from build123d import *

# Parameters (mm, degrees)
ESQUISSE1_W             = 9.3
ESQUISSE1_H             = 75
BOSS_EXTRU_1_DEPTH      = 6.5
ESQUISSE2_R             = 0.75
ENL_V_MAT_EXTRU_1_DEPTH = 4
ESQUISSE3_W             = 1.2
ESQUISSE3_H             = 67
ENL_V_MAT_EXTRU_2_DEPTH = 4
BOSS_EXTRU_2_DEPTH      = 0.6


with BuildPart() as part:
    # Esquisse1 → Boss.-Extru.1 (new body)
    with BuildSketch(Plane(origin=(0, 0, 0), x_dir=(1, 0, 0), z_dir=(0, 1, 0))):
        Rectangle(ESQUISSE1_W, ESQUISSE1_H)
    extrude(amount=BOSS_EXTRU_1_DEPTH)

    # Esquisse2 → Enlèv. mat.-Extru.1 (cut)
    with BuildSketch(Plane(origin=(0, 6.5, 0), x_dir=(1, 0, 0), z_dir=(0, 1, 0))):
        with Locations(Location((0, 35.5, 0), (0, 0, 270))):
            Circle(ESQUISSE2_R)
        with Locations(Location((0, -35.5, 0), (0, 0, 270))):
            Circle(ESQUISSE2_R)
    extrude(amount=-ENL_V_MAT_EXTRU_1_DEPTH, mode=Mode.SUBTRACT)

    # Esquisse3 → Enlèv. mat.-Extru.2 (cut)
    with BuildSketch(Plane(origin=(0, 6.5, 0), x_dir=(1, 0, 0), z_dir=(0, 1, 0))):
        Rectangle(ESQUISSE3_W, ESQUISSE3_H)
    extrude(amount=-ENL_V_MAT_EXTRU_2_DEPTH, mode=Mode.SUBTRACT)

    # Esquisse4 → Boss.-Extru.2 (add, symmetric)
    with BuildSketch(Plane(origin=(0, 0, 0), x_dir=(0, 0, -1), z_dir=(1, 0, 0))):
        Polygon((-26.491586963, 2.5), (-21.491586963, 2.5), (-21.491586963, 11), (-21.991586963, 11.5), (-21.991586963, 21.5), (-25.991586963, 21.5), (-25.991586963, 11.5), (-26.491586963, 11), align=None)
    extrude(amount=BOSS_EXTRU_2_DEPTH, both=True)


solid = part.part
Verification items for the finished model (mm, model axes). A direction names the side the tool comes from. Give positions to 0.01 mm unless a question says otherwise; leave off trailing zeros. Write each loop counter-clockwise with the first axis right and the second up, starting at its lowest first coordinate (ties: lowest second). Pieces come first, ordered by that corner, then holes. Notation, with made-up numbers: (55.25, -7.5) -> (73.25, -7.5) arc R11 ccw to (73.25, 13.5) -> close; hole circle Ø9 at (-2.75, -20.5). An arc over 180 degrees is marked (long way). Use CSV: the item, a comma, the result in double quotes.
(1) Sectioned sample at B-B (z = -35.5). Record the cut outline in (x, y).
Derived:
outline,"(-4.65, 0) -> (4.65, 0) -> (4.65, 6.5) -> (0.75, 6.5) -> (0.75, 2.5) -> (-0.75, 2.5) -> (-0.75, 6.5) -> (-4.65, 6.5) -> close"
(2) Set-up check for faces 4 (the cylindrical face through (0.225, 4.528, -34.785)), 5 (the flat face through (0, 17, 25.992)), 6 (the flat face through (0.6, 14, 24)): record each of +Z, -Z, +X, -X, +Y, -Y from which the full face is reachable in a straight line by a thin tool's end or side.
Derived:
face 4,"+Y"
face 5,"+Z, +X, -X, +Y"
face 6,"+Z, -Z, +X, +Y"
(3) Go/stop test with flat-tipped pins: pin 1 (1.5 mm diameter, centred on x = -2, z = -28, fed in from +Y); pin 2 (1 mm diameter, centred on x = 0, y = 8.5, fed in from +Z); pin 3 (3 mm diameter, centred on x = -2, y = 16.5, fed in from +Z); pin 4 (2 mm diameter, centred on x = -3, y = 12, fed in from +Z). Record where each tip stops, or that it passes through.
Derived:
pin 1,"stops at y = 6.5"
pin 2,"stops at z = 26.49"
pin 3,"stops at z = 25.99"
pin 4,"passes through"
(4) Sectioned sample at D-D (z = 12). Record the cut outline in (x, y), plus the area to 4 significant figures.
Derived:
outline,"(-4.65, 0) -> (4.65, 0) -> (4.65, 6.5) -> (0.6, 6.5) -> (0.6, 2.5) -> (-0.6, 2.5) -> (-0.6, 6.5) -> (-4.65, 6.5) -> close"
area,"55.65 mm^2"
(5) Release check for a two-part mould opening along X. For faces 1 (the flat face through (0, 2.5, 30)), 2 (the flat face through (-1, 6.5, -1)), 3 (the flat face through (4.65, 3, 1)) record: +X half, -X half, draft (parallel to the pull), parting line (faces both ways), or undercut.
Derived:
face 1,"undercut"
face 2,"draft"
face 3,"+X half"
(6) Sectioned sample at A-A (y = 3.5). Record the cut outline in (x, z).
Derived:
outline,"(-4.65, -37.5) -> (4.65, -37.5) -> (4.65, 37.5) -> (-4.65, 37.5) -> close; hole circle Ø1.5 at (0, -35.5); hole circle Ø1.5 at (0, 35.5); hole (-0.6, -33.5) -> (0.6, -33.5) -> (0.6, 21.49) -> (-0.6, 21.49) -> close; hole (-0.6, 26.49) -> (0.6, 26.49) -> (0.6, 33.5) -> (-0.6, 33.5) -> close"
(7) Sectioned sample at C-C (x = -2). Record the cut outline in (y, z), plus the area to 4 significant figures.
Derived:
outline,"(0, -37.5) -> (6.5, -37.5) -> (6.5, 37.5) -> (0, 37.5) -> close"
area,"487.5 mm^2"
(8) Material ranges on L1, parallel to X at y = 6.25, z = -24; L2, parallel to X at y = 3.9, z = 35.5; L3, parallel to Z at x = -0.25, y = 4.5, recorded low to high.
Derived:
L1,"x = -4.65 to -0.6, 0.6 to 4.65"
L2,"x = -4.65 to -0.75, 0.75 to 4.65"
L3,"z = -37.5 to -36.21, -34.79 to -33.5, 21.49 to 26.49, 33.5 to 34.79, 36.21 to 37.5"
